```python
from build123d import *

# Parameters (mm, degrees)
SKETCH1_R      = 40.5
SKETCH1_R_2    = 6.5
EXTRUDE1_DEPTH = 0.5


with BuildPart() as part:
    # Sketch1 → Extrude1 (new body)
    with BuildSketch(Plane.XY):
        with BuildLine():
            Line((-31.419788217, -53.5000001), (31.419788217, -53.5000001))
            ThreePointArc((31.419788217, -53.5000001), (42.551411722, -51.358337419), (52.093689717, -45.239130643))
            ThreePointArc((52.093689717, -45.239130643), (69.907481155, -0.240172639), (47.122602539, 42.457446655))
            ThreePointArc((47.122602539, 42.457446655), (41.424181091, 45.462448781), (35.066073476, 46.4999999))
            Line((35.066073476, 46.4999999), (-35.066073476, 46.4999999))
            ThreePointArc((-35.066073476, 46.4999999), (-41.425769339, 45.462104521), (-47.125508858, 42.456122536))
            ThreePointArc((-47.125508858, 42.456122536), (-69.908118584, -0.241920052), (-52.093134412, -45.239658724))
            ThreePointArc((-52.093134412, -45.239658724), (-42.551055918, -51.358479588), (-31.419788217, -53.5000001))
        make_face()
        Circle(SKETCH1_R, mode=Mode.SUBTRACT)
        with Locations((-44.917257263, 26.2)):
            Circle(SKETCH1_R_2, mode=Mode.SUBTRACT)
        with Locations((-36.024297356, -37.5)):
            Circle(SKETCH1_R_2, mode=Mode.SUBTRACT)
        with Locations((36.789094852, -36.75)):
            Circle(SKETCH1_R_2, mode=Mode.SUBTRACT)
        with Locations((52, 0)):
            Circle(SKETCH1_R_2, mode=Mode.SUBTRACT)
    extrude(amount=EXTRUDE1_DEPTH)


solid = part.part
```
Part model, mm, in its own coordinate system. Round coordinates to 2 decimals unless told otherwise and drop trailing zeros. Write each loop counter-clockwise with the first axis right and the second up, starting at its lowest first coordinate (ties: lowest second). Pieces come first, ordered by that corner, then holes. Notation, with made-up numbers: (-6, 27) -> (6, 27) arc R19 cw to (6, 43) -> close; hole circle Ø11 at (77.25, 56.5). An arc over 180 degrees is marked (long way). Return JSON: item names as keys, results as strings. Group by question number.
Q1. Mould opens along Y. For faces 1 (the cylindrical face through (-69.864, 0.456, 0.246)), 2 (the cylindrical face through (42.99, -34.8, 0.25)), 3 (the cylindrical face through (42.4, -51.42, 0.25)), 4 (the cylindrical face through (-41.34, 45.49, 0.25)) say: pulls with the +Y half, pulls with the -Y half, needs draft (parallel to the pull), parting line crosses it, or undercut.
Q2. Saw through at A-A on x = 0. Write the cut outline in (y, z).
Q3. Saw through at B-B on z = 0.35. Write the cut outline in (x, y), plus the area to 3 significant figures.
Q4. Pin check, flat tip, straight feed: pin 1 (11.5 mm diameter, centred on x = 52, y = 0, fed in from +Z). Stop position of the tip, or through.
Q5. Probe L1, parallel to X at y = -41.5, z = 0.3; L2, parallel to Y at x = 0, z = 0.3; L3, parallel to X at y = 4, z = 0.4. List the from-to ranges inside material, lowest first. Write a range as [from, to].
Q6. Saw through at C-C on y = -23.5. Write the cut outline in (x, z), plus the area to 3 significant figures.
Q7. Saw through at D-D on y = 28. Write the cut outline in (x, z), plus the area to 3 significant figures.
Answer:
{
 "1": {"face 1": "parting line crosses it", "face 2": "undercut", "face 3": "pulls with the -Y half", "face 4": "pulls with the +Y half"},
 "2": {"outline": "(-53.5, 0) -> (-40.5, 0) -> (-40.5, 0.5) -> (-53.5, 0.5) -> close; (40.5, 0) -> (46.5, 0) -> (46.5, 0.5) -> (40.5, 0.5) -> close"},
 "3": {"outline": "(-52.09, -45.24) arc R30 ccw to (-31.42, -53.5) -> (31.42, -53.5) arc R30 ccw to (52.09, -45.24) arc R57.6 ccw to (47.12, 42.46) arc R20 ccw to (35.07, 46.5) -> (-35.07, 46.5) arc R20 ccw to (-47.13, 42.46) arc R57.6 ccw to start; hole circle Ø13 at (-44.92, 26.2); hole circle Ø13 at (-36.02, -37.5); hole circle Ø81 at (0, 0); hole circle Ø13 at (36.79, -36.75); hole circle Ø13 at (52, 0)", "area": "6,600 mm2"},
 "4": {"pin 1": "through"},
 "5": {"L1": "[-55.69, -41.15], [-30.9, 32.35], [41.23, 55.69]", "L2": "[-53.5, -40.5], [40.5, 46.5]", "L3": "[-69.51, -40.3], [40.3, 46.88], [57.12, 69.51]"},
 "6": {"outline": "(-66.42, 0) -> (-32.98, 0) -> (-32.98, 0.5) -> (-66.42, 0.5) -> close; (32.98, 0) -> (66.42, 0) -> (66.42, 0.5) -> (32.98, 0.5) -> close", "area": "33.4 mm2"},
 "7": {"outline": "(-60.62, 0) -> (-51.16, 0) -> (-51.16, 0.5) -> (-60.62, 0.5) -> close; (-38.67, 0) -> (-29.26, 0) -> (-29.26, 0.5) -> (-38.67, 0.5) -> close; (29.26, 0) -> (60.62, 0) -> (60.62, 0.5) -> (29.26, 0.5) -> close", "area": "25.1 mm2"}
}
